Could you check a few things on this drawing? It's one solid part, dimensions in mm from its lowest x, y, z. Give positions to 0.01 mm unless a question says otherwise; leave off trailing zeros. Loops run counter-clockwise (first coordinate to the right, second up) from the corner with the lowest first, then second, coordinate; pieces in that order, holes last.
Q1. Suppose I cut it at B-B (x = 67). List the corners of the cut face in (y, z) for me (1 decimal).
Q2. I'm going to push a flat-ended pin straight in: P1, Ø10.5, axis at x = 41.98, z = 33.86, coming from the +Y side. Where does the tip first touch, or does it pass through?
Q3. Suppose I cut it at C-C (y = 7). List the corners of the cut face in (x, z) for me (1 decimal).
Q4. I need wall thicknesses on probe 1 along X at (y, z) = (1, 35.5) (1 decimal); probe 2 along X at (y, z) = (8.75, 32.5) (1 decimal); probe 3 along Z at (x, y) = (80, 9) (1 decimal). Which ranges of each line are inside material? Lowest first, please.
Q5. Suppose I cut it at A-A (z = 26). List the corners of the cut face in (x, y) for me (1 decimal).
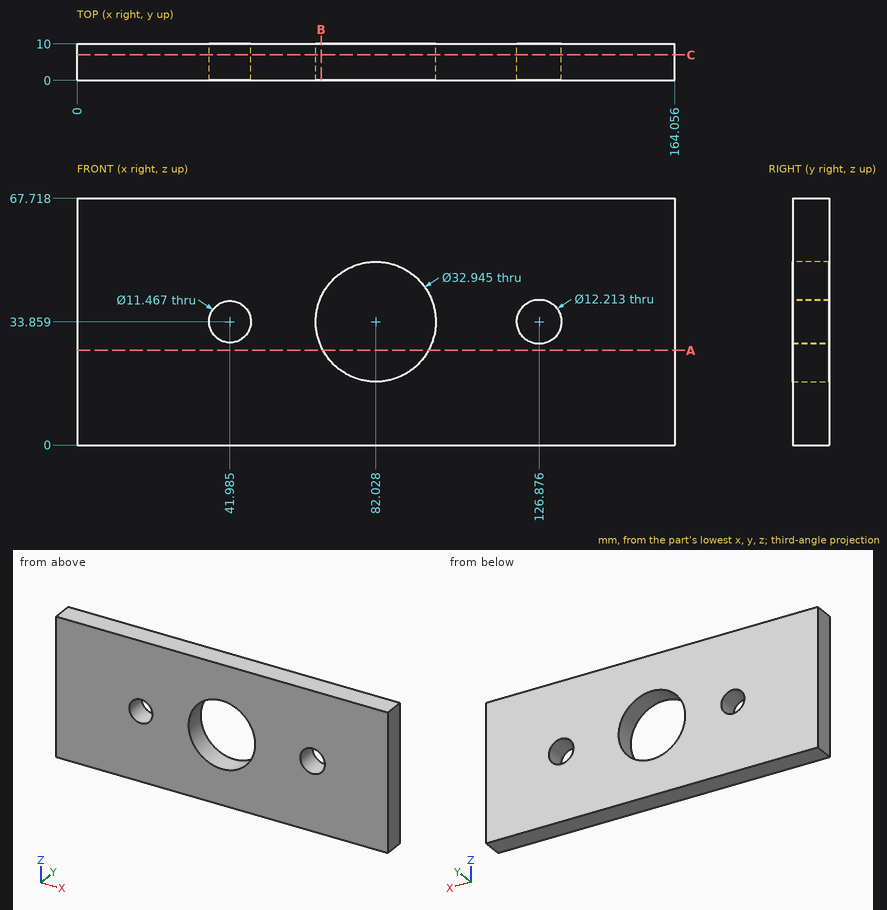
Solutions:
1. outline: (0, 0) - (10, 0) - (10, 27.1) - (0, 27.1) - close; (0, 40.6) - (10, 40.6) - (10, 67.7) - (0, 67.7) - close
2. P1: passes through
3. outline: (0, 0) - (164.1, 0) - (164.1, 67.7) - (0, 67.7) - close; hole circle Ø11.5 at (42, 33.9); hole circle Ø32.9 at (82, 33.9); hole circle Ø12.2 at (126.9, 33.9)
4. probe 1: x = 0 to 36.5, 47.5 to 65.6, 98.4 to 121, 132.8 to 164.1
4. probe 2: x = 0 to 36.4, 47.6 to 65.6, 98.4 to 120.9, 132.8 to 164.1
4. probe 3: z = 0 to 17.5, 50.2 to 67.7
5. outline: (0, 0) - (67.6, 0) - (67.6, 10) - (0, 10) - close; (96.5, 0) - (164.1, 0) - (164.1, 10) - (96.5, 10) - close
